The figure shows three views and two pictorial views of one solid part (mm, origin at its lowest corner). Answer the questions. Give positions to 0.01 mm unless a question says otherwise; leave off trailing zeros. Loops run counter-clockwise (first coordinate to the right, second up) from the corner with the lowest first, then second, coordinate; pieces in that order, holes last. Notation, with made-up numbers: (42.25, -25.5) -> (89.25, -25.5) arc R10 cw to (89.25, -15.5) -> close; hole circle Ø9 at (-25.75, 37.25). An arc over 180 degrees is marked (long way). One line per item, written item: value. Start each with the question number.
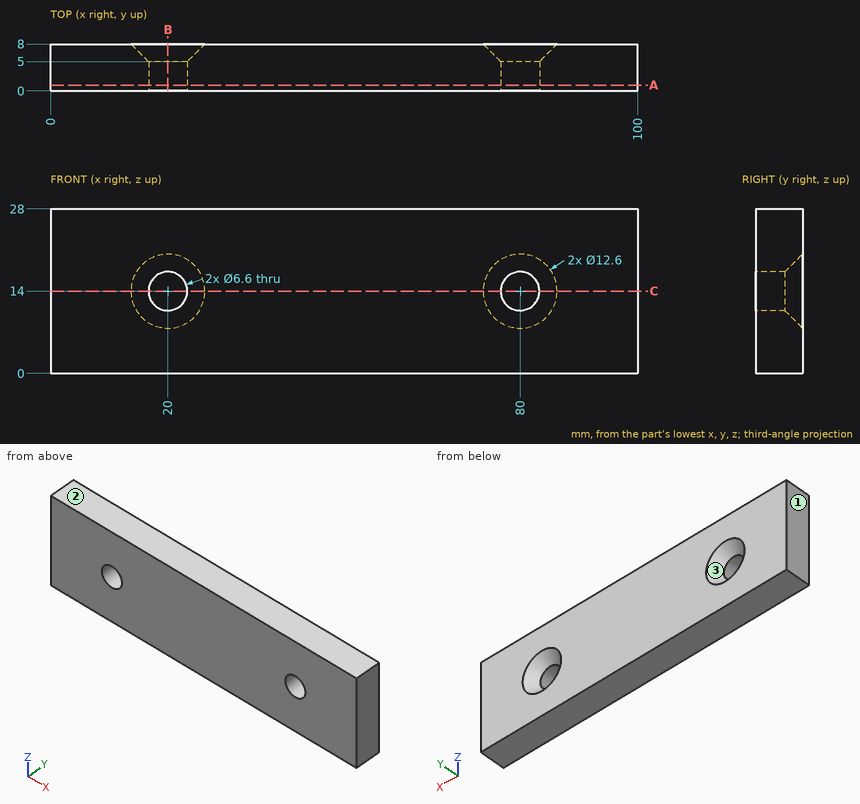
Item 1: Section A-A, the plane y = 1 is taken. Determine the outline of the cut face in (x, z), plus the area to 3 significant figures.
Item 2: Section B-B, the plane x = 20 is taken. Determine the outline of the cut face in (y, z).
Item 3: A flat-ended cylindrical pin translates along its axis: pin 1 (7.5 mm diameter, centred on x = 80, z = 14, fed in from +Y). Find the tip coordinate at first contact, or state that the pin passes through.
Item 4: Section C-C, the plane z = 14 is taken. Determine the outline of the cut face in (x, y), plus the area to 3 significant figures.
Item 5: Determine the mould class of the marked faces 1, 2 and 3 for opening direction Z: pulls with the +Z half, pulls with the -Z half, needs draft (parallel to the pull), parting line crosses it, or undercut.
Item 6: Consider L1, parallel to X at y = 2.45, z = 14; L2, parallel to Z at x = 80, y = 2.8; L3, parallel to X at y = 7, z = 13. Determine where each line is inside the solid, lowest interval first. Write a range as [from, to].
Computed values:
1. outline: (0, 0) -> (100, 0) -> (100, 28) -> (0, 28) -> close; hole circle Ø6.6 at (20, 14); hole circle Ø6.6 at (80, 14)
1. area: 2,730 mm²
2. outline: (0, 0) -> (8, 0) -> (8, 7.7) -> (5, 10.7) -> (0, 10.7) -> close; (0, 17.3) -> (5, 17.3) -> (8, 20.3) -> (8, 28) -> (0, 28) -> close
3. pin 1: y = 5.45
4. outline: (0, 0) -> (16.7, 0) -> (16.7, 5) -> (13.7, 8) -> (0, 8) -> close; (23.3, 0) -> (76.7, 0) -> (76.7, 5) -> (73.7, 8) -> (26.3, 8) -> (23.3, 5) -> close; (83.3, 0) -> (100, 0) -> (100, 8) -> (86.3, 8) -> (83.3, 5) -> close
4. area: 676 mm²
5. face 1: needs draft
5. face 2: pulls with the +Z half
5. face 3: undercut
6. L1: [0, 16.7], [23.3, 76.7], [83.3, 100]
6. L2: [0, 10.7], [17.3, 28]
6. L3: [0, 14.8], [25.2, 74.8], [85.2, 100]
